Verification items for this drawing (mm, ordinates from the low corner). Round coordinates to 2 decimals unless told otherwise and drop trailing zeros. Write each loop counter-clockwise with the first axis right and the second up, starting at its lowest first coordinate (ties: lowest second). Pieces come first, ordered by that corner, then holes. Notation, with made-up numbers: (-22, 73.25) -> (-8, 73.25) arc R33 cw to (-8, 102.25) -> close; hole circle Ø9 at (-4.75, -25.5). An arc over 180 degrees is marked (long way). One line per question, with ' | ' between items.
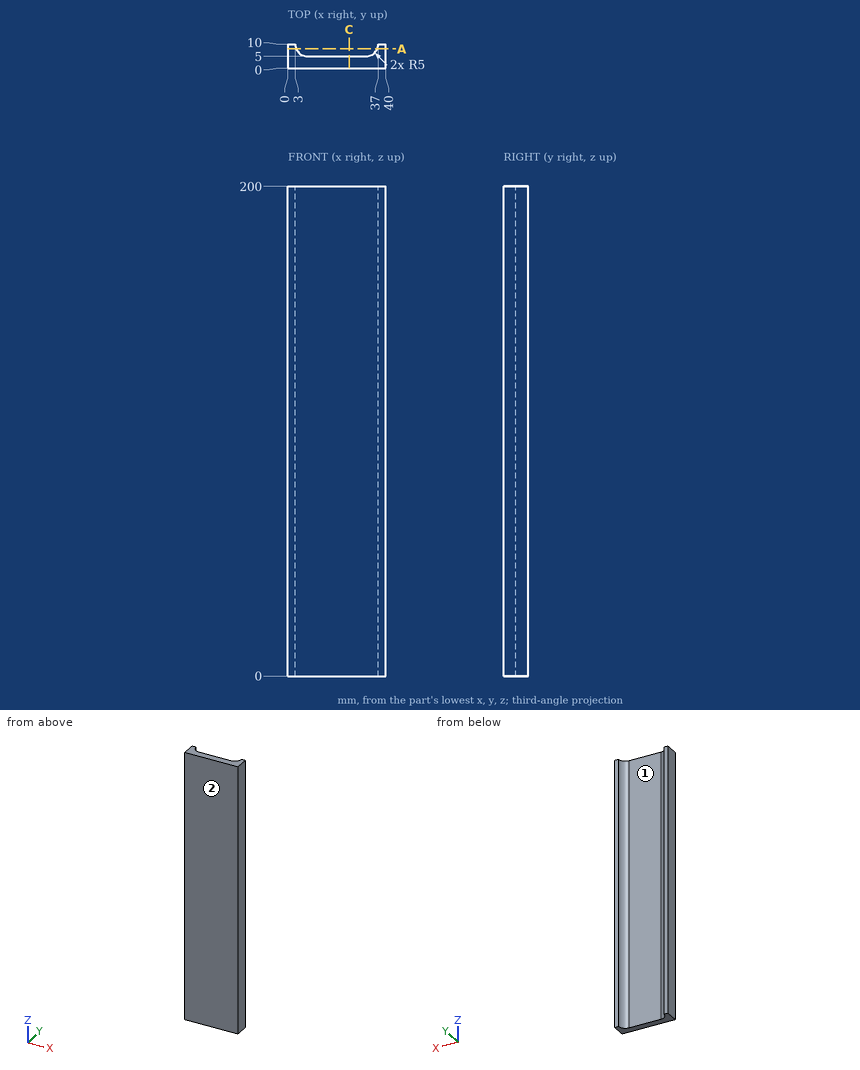
(1) Material ranges on line 1 (Y direction, x = 15, z = 126); line 2 (X direction, y = 5.5, z = 42) (1 decimal); line 3 (Y direction, x = 33, z = 165), recorded low to high.
Resolved:
line 1: y = 0 to 5 | line 2: x = 0 to 5.8, 34.2 to 40 | line 3: y = 0 to 5.1
(2) Sectioned sample at C-C on x = 25. Record the cut outline in (y, z), then the cut area to 3 significant figures.
Resolved:
outline: (0, 0) -> (5, 0) -> (5, 200) -> (0, 200) -> close | area: 1,000 mm2
(3) Sectioned sample at A-A on y = 8. Record the cut outline in (x, z), then the cut area to 3 significant figures.
Resolved:
outline: (0, 0) -> (3.42, 0) -> (3.42, 200) -> (0, 200) -> close; (36.58, 0) -> (40, 0) -> (40, 200) -> (36.58, 200) -> close | area: 1,370 mm2
(4) Go/stop test with flat-tipped pins: pin 1 (4 mm diameter, centred on y = 7, z = 112.5, fed in from -X); pin 2 (19 mm diameter, centred on x = 14.5, z = 59.5, fed in from +Y). Record where each tip stops, or that it passes through.
Resolved:
pin 1: stops at x = 0 | pin 2: stops at y = 6
(5) Draft check along X on the marked faces 1 and 2. Enter one of: +X half, -X half, draft (parallel to the pull), parting line (faces both ways), or undercut.
Resolved:
face 1: undercut | face 2: draft
